from build123d import *

# Parameters (mm, degrees)
EXTRUDE_1_DEPTH              = 10
HOLE_WIZARD_M3_2_D           = 2.5
HOLE_WIZARD_M3_2_CSINK_D     = 2.55
HOLE_WIZARD_M3_2_CSINK_ANGLE = 90
SKETCH_15_W                  = 10
SKETCH_15_H                  = 10
EXTRUDE_2_DEPTH              = 5
HOLE_WIZARD_M3_1_D           = 2.5
HOLE_WIZARD_M3_1_CSINK_D     = 2.55
HOLE_WIZARD_M3_1_CSINK_ANGLE = 90
SKETCH_21_W                  = 8.291796068
SKETCH_21_H                  = 10
CUT_EXTRUDE_2_DEPTH          = 5
SKETCH_23_R                  = 1.65
CUT_EXTRUDE_3_DEPTH          = 10
SKETCH_24_R                  = 1.65
CUT_EXTRUDE_4_DEPTH          = 10


with BuildPart() as part:
    # 草图1 → 凸台-拉伸1 (new body)
    with BuildSketch(Plane(origin=(0, 0, 0), x_dir=(1, 0, 0), z_dir=(0, 1, 0))):
        with BuildLine():
            Line((0, 0), (0, -10))
            ThreePointArc((0, -10), (-5, -15), (0, -20))
            Line((0, -20), (0, -30))
            Line((0, -30), (-2, -30))
            Line((-2, -30), (-2, -21.708203932))
            ThreePointArc((-2, -21.708203932), (-7, -15), (-2, -8.291796068))
            Line((-2, -8.291796068), (-2, 0))
            Line((-2, 0), (0, 0))
        make_face()
    extrude(amount=EXTRUDE_1_DEPTH)

    # M3 螺纹孔的螺纹孔钻头2 (through all)
    with Locations(Plane.ZY.offset(7)):
        with Locations((15, 5)):
            CounterSinkHole(HOLE_WIZARD_M3_2_D / 2, HOLE_WIZARD_M3_2_CSINK_D / 2, counter_sink_angle=HOLE_WIZARD_M3_2_CSINK_ANGLE)

    # 草图15 → 凸台-拉伸2 (add)
    with BuildSketch(Plane(origin=(0, 0, 0), x_dir=(0, 0, -1), z_dir=(1, 0, 0))):
        with Locations((-5, 5)):
            Rectangle(SKETCH_15_W, SKETCH_15_H)
        with Locations((-25, 5)):
            Rectangle(SKETCH_15_W, SKETCH_15_H)
    extrude(amount=EXTRUDE_2_DEPTH)

    # M3 螺纹孔的螺纹孔钻头1 (through all)
    with Locations(Plane(origin=(5, 0, 0), x_dir=(0, 0, -1), z_dir=(1, 0, 0))):
        with Locations((-5, 5), (-25, 5)):
            CounterSinkHole(HOLE_WIZARD_M3_1_D / 2, HOLE_WIZARD_M3_1_CSINK_D / 2, counter_sink_angle=HOLE_WIZARD_M3_1_CSINK_ANGLE)

    # 草图21 → 切除-拉伸2 (cut)
    with BuildSketch(Plane.ZY.offset(2)):
        with Locations((4.145898034, 5)):
            Rectangle(SKETCH_21_W, SKETCH_21_H)
        with Locations((25.854101966, 5)):
            Rectangle(SKETCH_21_W, SKETCH_21_H)
    extrude(amount=-CUT_EXTRUDE_2_DEPTH, mode=Mode.SUBTRACT)

    # 草图23 → 切除-拉伸3 (cut)
    with BuildSketch(Plane.ZY.offset(-3)):
        with Locations((25, 5)):
            Circle(SKETCH_23_R)
        with Locations((5, 5)):
            Circle(SKETCH_23_R)
    extrude(amount=-CUT_EXTRUDE_3_DEPTH, mode=Mode.SUBTRACT)

    # 草图24 → 切除-拉伸4 (cut)
    with BuildSketch(Plane.ZY.offset(7)):
        with Locations((15, 5)):
            Circle(SKETCH_24_R)
    extrude(amount=-CUT_EXTRUDE_4_DEPTH, mode=Mode.SUBTRACT)


solid = part.part
Geometry check sheet. Reference: the model listing, model coordinates, mm. A direction names the side the tool comes from. Give positions to 0.01 mm unless a question says otherwise; leave off trailing zeros. Loops run counter-clockwise (first coordinate to the right, second up) from the corner with the lowest first, then second, coordinate; pieces in that order, holes last.
(1) Section check A-A on x = 3.75. Record the cut outline in (y, z).
From the geometry:
outline: (0, 0) - (10, 0) - (10, 10) - (0, 10) - close; (0, 20) - (10, 20) - (10, 30) - (0, 30) - close; hole circle Ø3.3 at (5, 5); hole circle Ø3.3 at (5, 25)
(2) Section check D-D on x = -2.5. Record the cut outline in (y, z), then the cut area to 3 significant figures.
From the geometry:
outline: (0, 8.46) - (10, 8.46) - (10, 10.67) - (0, 10.67) - close; (0, 19.33) - (10, 19.33) - (10, 21.54) - (0, 21.54) - close
area: 44.2 mm2
(3) Section check B-B on z = 15. Record the cut outline in (x, y).
From the geometry:
outline: (-7, 0) - (-5, 0) - (-5, 3.35) - (-7, 3.35) - close; (-7, 6.65) - (-5, 6.65) - (-5, 10) - (-7, 10) - close
(4) Thickness scan on L1, parallel to Y at x = -5.65, z = 15; L2, parallel to Z at x = 2.5, y = 1.75; L3, parallel to X at y = 7.75, z = 6.25. Record the ranges inside material, lowest first.
From the geometry:
L1: y = 0 to 3.35, 6.65 to 10
L2: z = 8.29 to 10, 20 to 21.71
L3: x = 3 to 5
(5) Depth check by flat-ended pin: pin 1 Ø1.5 at (y, z) = (5.5, 11.5) entering from -X; pin 2 Ø3 at (x, y) = (-5, 2) entering from +Z; pin 3 Ø4 at (x, y) = (-3.5, 7) entering from +Z. Enter the tip coordinate at first touch or a pass-through.
From the geometry:
pin 1: stops at x = -6.44
pin 2: stops at z = 21.06
pin 3: stops at z = 21.71
(6) Set-up check for faces 1 (the flat face through (3, 5, 3)), 2 (the flat face through (0, 5, 21.708)), 3 (the flat face through (5, 7, 25)), 4 (the flat face through (2, 5, 20)): record each of +Z, -Z, +X, -X, +Y, -Y from which the full face is reachable in a straight line by a thin tool's end or side.
From the geometry:
face 1: -Z, -X, +Y, -Y
face 2: +Z, -X, +Y, -Y
face 3: +Z, -Z, +X, +Y, -Y
face 4: +X, +Y, -Y
(7) Release check for a two-part mould opening along Y. For faces 5 (the cylindrical face through (-5.876, 6.115, 13.784)), 6 (the flat face through (-2.8, 0, 10.6)), 7 (the flat face through (0, 5, 8.292)), 8 (the flat face through (-2.8, 10, 10.6)) record: released by +Y, released by -Y, zero draft, split by the parting line, or undercut.
From the geometry:
face 5: undercut
face 6: released by -Y
face 7: zero draft
face 8: released by +Y
(8) Section check C-C on y = 5. Record the cut outline in (x, z).
From the geometry:
outline: (-6.8, 13.35) arc R7 ccw to (-2, 8.29) - (3, 8.29) - (3, 6.65) - (5, 6.65) - (5, 10) - (0, 10) arc R5 cw to (-4.72, 13.35) - close; (-6.8, 16.65) - (-4.72, 16.65) arc R5 cw to (0, 20) - (5, 20) - (5, 23.35) - (3, 23.35) - (3, 21.71) - (-2, 21.71) arc R7 ccw to start; (3, 0) - (5, 0) - (5, 3.35) - (3, 3.35) - close; (3, 26.65) - (5, 26.65) - (5, 30) - (3, 30) - close
